Check sheet for the modelled part. Datum: model origin and axes. Units: mm. A direction names the side the tool comes from. Give positions to 0.01 mm unless a question says otherwise; leave off trailing zeros. Loops run counter-clockwise (first coordinate to the right, second up) from the corner with the lowest first, then second, coordinate; pieces in that order, holes last. Notation, with made-up numbers: M 21.25,76.25 L 77.25,76.25 A16 cw 77.25,85.25 Z; hole C 32.25,-35 d9. An arc over 180 degrees is marked long. Use one line per item in the form item = value.
from build123d import *

# Parameters (mm, degrees)
SKETCH1_W           = 20
SKETCH1_H           = 120
BOSS_EXTRUDE1_DEPTH = 30
SKETCH2_W           = 40
SKETCH2_H           = 40
BOSS_EXTRUDE2_DEPTH = 20
FILLET1_R           = 10


with BuildPart() as part:
    # Sketch1 → Boss-Extrude1 (new body)
    with BuildSketch(Plane.XY):
        with Locations((-20, -60)):
            Rectangle(SKETCH1_W, SKETCH1_H)
    extrude(amount=BOSS_EXTRUDE1_DEPTH)

    # Sketch2 → Boss-Extrude2 (add)
    with BuildSketch(Plane.XY):
        with Locations((-10, -100)):
            Rectangle(SKETCH2_W, SKETCH2_H)
    extrude(amount=-BOSS_EXTRUDE2_DEPTH)

    # Fillet1
    fillet1_edges = [part.edges().sort_by_distance(p)[0] for p in [
        (10, -80, -10),
        (-20, 0, 30),
    ]]
    fillet(fillet1_edges, radius=FILLET1_R)


solid = part.part
1) Depth check by flat-ended pin: pin 1 Ø9 at (y, z) = (-43, 20) entering from +X; pin 2 Ø12 at (x, z) = (-22, -12) entering from +Y; pin 3 Ø10 at (x, y) = (1, -106.5) entering from +Z; pin 4 Ø6 at (x, z) = (-6.5, 14.5) entering from +Y. Enter the tip coordinate at first touch or a pass-through.
Evaluation:
pin_1 = -10
pin_2 = -80
pin_3 = 0
pin_4 = through
2) Set-up check for faces 1 (the face through (0, -100, 0)), 2 (the face through (-19.86, -3.01, 27.15)), 3 (the face through (-20, -39, 0)): record each of +Z, -Z, +X, -X, +Y, -Y from which the full face is reachable in a straight line by a thin tool's end or side.
Evaluation:
face_1 = +Z, +X, +Y, -Y
face_2 = +Z, +X, -X, +Y
face_3 = -Z, +X, -X, +Y
3) Section check D-D (y = -108.5). Record the cut outline in (x, z), then the cut area to 3 significant figures.
Evaluation:
outline = M -30,-20 L 10,-20 L 10,0 L -10,0 L -10,30 L -30,30 Z
area = 1,400 mm^2
4) Section check B-B (y = -84). Record the cut outline in (x, z).
Evaluation:
outline = M -30,-20 L 8,-20 L 8,0 L -10,0 L -10,30 L -30,30 Z
5) Scan lines: line 1 (Y direction, x = -25, z = -6.5); line 2 (X direction, y = -84.5, z = 1.5); line 3 (Z direction, x = -21.5, y = -55). Record each from-to range of solid material in increasing order.
Evaluation:
line_1 = -120 to -80
line_2 = -30 to -10
line_3 = 0 to 30
6) Section check C-C (z = -15). Record the cut outline in (x, y).
Evaluation:
outline = M -30,-120 L 10,-120 L 10,-90 A10 ccw 0,-80 L -30,-80 Z
7) Section check A-A (x = -14.5). Record the cut outline in (y, z).
Evaluation:
outline = M -120,-20 L -80,-20 L -80,0 L 0,0 L 0,20 A10 ccw -10,30 L -120,30 Z
